For this review, use the dimensioned drawing (mm, ordinates from the lowest corner) and the shaded views. A direction names the side the tool comes from. Coordinates: 2 decimals unless noted, no trailing zeros. Order: outer loops, then holes, each group sorted by start corner. A loop starts at its lowest first (then second) coordinate and runs counter-clockwise, first axis right, second up. Notation, with made-up numbers: M 53,-27.5 L 78,-27.5 A22 cw 78,-14.5 Z; hole C -37,37.5 d5. An arc over 180 degrees is marked long. Answer in a Markdown table with one row per item.
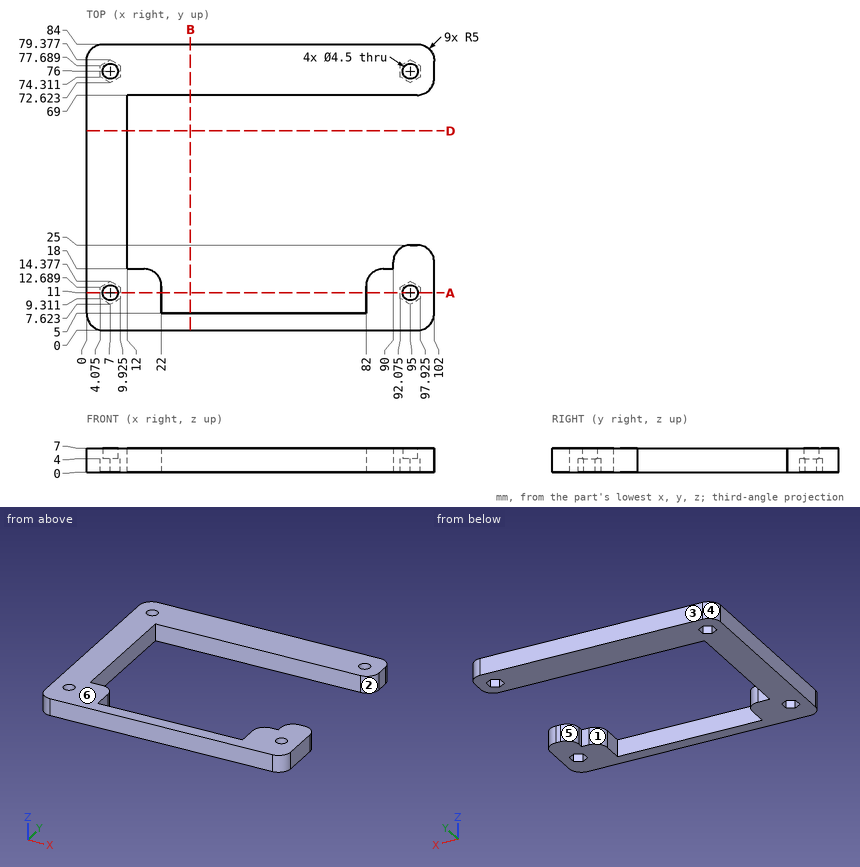
(1) For the marked faces 1, 2 and 3, list the 3-axis set-ups (+Z, -Z, +X, -X, +Y, -Y) from which the entire face can be reached by the end or side of a thin tool; tool diameter is ignored.
Return value:
| item | result |
|---|---|
| face 1 | +Z, -Z |
| face 2 | +Z, -Z, +X |
| face 3 | +Z, -Z, +X, -X, +Y |
(2) For line 1 along Y through (x, z) = (95, 6.2); line 2 along X through (y, z) = (11, 5.7); line 3 along X through (y, z) = (76, 5.05), list the stretches that pass through material, from the lowest coordinate up. Write a range as from..to.
Return value:
| item | result |
|---|---|
| line 1 | y = 0..8.75, 13.25..25, 69..73.75, 78.25..84 |
| line 2 | x = 0..4.75, 9.25..22, 82..92.75, 97.25..102 |
| line 3 | x = 0..4.75, 9.25..92.75, 97.25..102 |
(3) Add section D-D, the plane y = 58.5. Give the boundary of the cut face in (x, z), and give its area (3 significant figures).
Return value:
| item | result |
|---|---|
| outline | M 0,0 L 12,0 L 12,7 L 0,7 Z |
| area | 84.0 mm2 |
(4) Add section B-B, the plane x = 30.5. Give the boundary of the cut face in (y, z), and give its area (3 significant figures).
Return value:
| item | result |
|---|---|
| outline | M 0,0 L 5,0 L 5,7 L 0,7 Z; M 69,0 L 84,0 L 84,7 L 69,7 Z |
| area | 140 mm2 |
(5) Draft analysis for pull direction X (two halves, no side actions). For the marked faces 4, 5 and 6, state which applies: pulls with the +X half, pulls with the -X half, needs draft (parallel to the pull), parting line crosses it, or undercut.
Return value:
| item | result |
|---|---|
| face 4 | pulls with the -X half |
| face 5 | undercut |
| face 6 | needs draft |
(6) Add section A-A, the plane y = 11. Give the number of separate pieces and of enclosed holes in the cut face, and give its area (3 significant figures).
Return value:
| item | result |
|---|---|
| separate pieces | 4 |
| enclosed holes | 0 |
| area | 220 mm2 |
